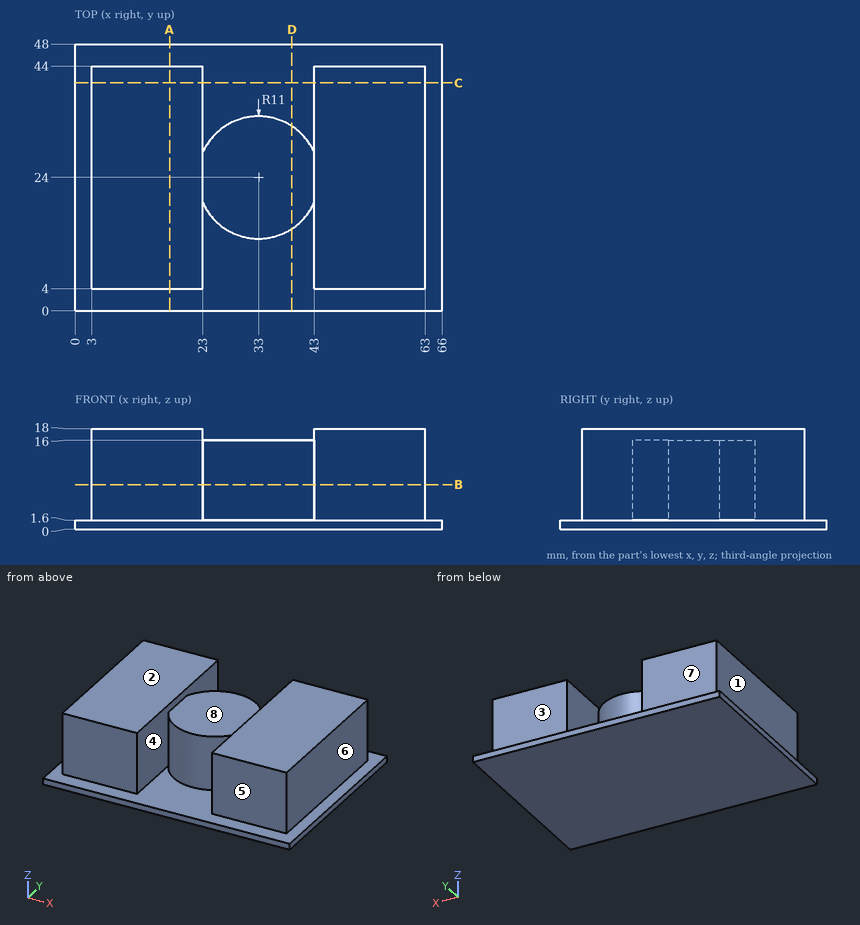
Could you check a few things on this drawing? It's one solid part, dimensions in mm from its lowest x, y, z. A direction names the side the tool comes from. Round coordinates to 2 decimals unless told otherwise and drop trailing zeros. Write each loop counter-clockwise with the first axis right and the second up, starting at its lowest first coordinate (ties: lowest second). Pieces come first, ordered by that corner, then holes.
Q1. Which directions (+Z, -Z, +X, -X, +Y, -Y) give clear straight access to the entire face, cutting with the end or side of a thin tool? Please do the marked faces 1, 2, 3, 4 and 5.
Q2. Will these pins go through, and if not, where does the flat tip stop? P1, Ø1.5, axis at x = 21, z = 8, coming from the +Y side; P2, Ø8, axis at x = 15.5, z = 10.5, coming from the -Y side; P3, Ø5, axis at y = 32.5, z = 12.5, coming from the +X side.
Q3. Please list where these lines run through material, in increasing order: probe 1 along X at (y, z) = (9.5, 14.5); probe 2 along X at (y, z) = (15.5, 2); probe 3 along X at (y, z) = (15, 8).
Q4. If we section it at D-D on x = 39: Write out the boundary of the cut face in (y, z), plus the area to 3 significant figures.
Q5. If we section it at A-A on x = 17: Write out the boundary of the cut face in (y, z).
Q6. If we mould it in two halves opening along X, with no side actions, what happens to the marked faces 6, 7 and 8? For each: +X half, -X half, draft (parallel to the pull), parting line (faces both ways), or undercut.
Q7. If we section it at B-B on z = 8: Write out the boundary of the cut face in (x, y).
Q8. If we section it at C-C on y = 41: Write out the boundary of the cut face in (x, z), plus the area to 3 significant figures.
Answer below:
1. face 1: +Z, -X, +Y, -Y
1. face 2: +Z, +X, -X, +Y, -Y
1. face 3: +Z, +X, -X, +Y
1. face 4: +Z
1. face 5: +Z, +X, -X, -Y
2. P1: stops at y = 44
2. P2: stops at y = 4
2. P3: stops at x = 63
3. probe 1: x = 3 to 23, 43 to 63
3. probe 2: x = 3 to 23, 26.02 to 39.98, 43 to 63
3. probe 3: x = 3 to 23, 26.68 to 39.32, 43 to 63
4. outline: (0, 0) - (48, 0) - (48, 1.6) - (33.22, 1.6) - (33.22, 16) - (14.78, 16) - (14.78, 1.6) - (0, 1.6) - close
4. area: 342 mm2
5. outline: (0, 0) - (48, 0) - (48, 1.6) - (44, 1.6) - (44, 18) - (4, 18) - (4, 1.6) - (0, 1.6) - close
6. face 6: +X half
6. face 7: draft
6. face 8: undercut
7. outline: (3, 4) - (23, 4) - (23, 19.42) arc R11 ccw to (43, 19.42) - (43, 4) - (63, 4) - (63, 44) - (43, 44) - (43, 28.58) arc R11 ccw to (23, 28.58) - (23, 44) - (3, 44) - close
8. outline: (0, 0) - (66, 0) - (66, 1.6) - (63, 1.6) - (63, 18) - (43, 18) - (43, 1.6) - (23, 1.6) - (23, 18) - (3, 18) - (3, 1.6) - (0, 1.6) - close
8. area: 762 mm2
